The listing builds one solid part. Answer for the finished solid, in the listing's coordinates (mm). A direction names the side the tool comes from. Give positions to 0.01 mm unless a question says otherwise; leave off trailing zeros. Loops run counter-clockwise (first coordinate to the right, second up) from the corner with the lowest first, then second, coordinate; pieces in that order, holes last. Notation, with made-up numbers: M -9,73 L 1,73 A34 cw 1,107 Z; hole C 42,88 d9. An arc over 180 degrees is marked long. Use one line per item in the form item = value. Start each with the question number.
1. The part is cut by section A-A (x = 402.5). Write down the section's boundary in (y, z), and give its area (3 significant figures).
2. Straight lines are drawn through the part: line 1 (X direction, y = 24.15, z = 0); line 2 (Z direction, x = 27, y = 1); line 3 (Z direction, x = -320, y = -2.5). For each, find the intervals that lie inside material, in ascending order. Write a range as from..to.
3. Each of these flat-tipped pins is pushed along its axis until it touches: pin 1 Ø3 at (x, z) = (-263.5, -5) entering from +Y; pin 2 Ø10.5 at (x, y) = (167, -2) entering from +Z; pin 3 Ø4 at (x, z) = (342.5, 10.5) entering from +Y. Where does it stop, or does it pass through?
4. The mould has two halves that part along Y. Classify faces 1 (the face through (-515, -13, -20)), 2 (the face through (7.2, -22.2, -11.5)), 3 (the face through (165.63, 6.31, -20.03)): released by +Y, released by -Y, zero draft, split by the parting line, or undercut.
5. For faces 4 (the face through (515, -13, -20)), 5 (the face through (120, -19, -10)), 6 (the face through (210, -19, -10)), determine the directions among +Z, -Z, +X, -X, +Y, -Y from which every point of the face is accessible in a straight line to the end or side of a thin tool.
from build123d import *

# Parameters (mm, degrees)
SKETCH1_R                     = 25
SKETCH1_R_2                   = 23
EXTRUDE_THIN1_DEPTH           = 515
EXTRUDE_THIN2_START           = 210
SKETCH1_3_R                   = 25
SKETCH1_3_R_2                 = 21
EXTRUDE_THIN2_DEPTH           = 90
CUT_EXTRUDE1_START            = 24.54
CUT_EXTRUDE1_DEPTH            = 492.672165684
CUT_EXTRUDE2_START            = -24.54
CUT_EXTRUDE2_DEPTH            = 492.672165793
CUT_EXTRUDE3_START            = -24.54
CUT_EXTRUDE3_DEPTH            = 492.672165793
CUT_EXTRUDE4_START            = 24.54
CUT_EXTRUDE4_DEPTH            = 492.672165793
M_0_295_DIAMETER_HOLE3_REACH  = 519.981
M_0_295_DIAMETER_HOLE3_BORE_R = 3.7465
M_0_295_DIAMETER_HOLE4_REACH  = 519.981
M_0_295_DIAMETER_HOLE4_BORE_R = 3.7465
M_0_295_DIAMETER_HOLE5_REACH  = 519.981
M_0_295_DIAMETER_HOLE5_BORE_R = 3.7465
M_0_295_DIAMETER_HOLE6_REACH  = 519.981
M_0_295_DIAMETER_HOLE6_BORE_R = 3.7465
CHAMFER1_SIZE                 = 0.5


with BuildPart() as part:
    # Sketch1 → Extrude-Thin1 (new, symmetric)
    with BuildSketch(Plane(origin=(0, 0, 0), x_dir=(0, 0, -1), z_dir=(1, 0, 0))):
        Circle(SKETCH1_R)
        Circle(SKETCH1_R_2, mode=Mode.SUBTRACT)
    extrude(amount=EXTRUDE_THIN1_DEPTH, both=True)

    # Sketch1<3> → Extrude-Thin2 (add)
    with BuildSketch(Plane(origin=(0, 0, 0), x_dir=(0, 0, -1), z_dir=(1, 0, 0)).offset(EXTRUDE_THIN2_START)):
        Circle(SKETCH1_3_R)
        Circle(SKETCH1_3_R_2, mode=Mode.SUBTRACT)
    extrude(amount=-EXTRUDE_THIN2_DEPTH)

    # Sketch3 → Cut-Extrude1 (cut, through all)
    with BuildSketch(Plane(origin=(0, 0, 0), x_dir=(1, 0, 0), z_dir=(0, 1, 0)).offset(CUT_EXTRUDE1_START)):
        with BuildLine():
            Line((-491.7775, -17.4725), (-458.1225, -17.4725))
            ThreePointArc((-458.1225, -17.4725), (-440.65, 0), (-458.1225, 17.4725))
            Line((-458.1225, 17.4725), (-491.7775, 17.4725))
            ThreePointArc((-491.7775, 17.4725), (-509.25, 0), (-491.7775, -17.4725))
        make_face()
    extrude(amount=CUT_EXTRUDE1_DEPTH, mode=Mode.SUBTRACT)

    # Sketch8 → Cut-Extrude2 (cut, through all)
    with BuildSketch(Plane.XY.offset(CUT_EXTRUDE2_START)):
        with BuildLine():
            Line((-272.5275, -17.4725), (-238.8725, -17.4725))
            ThreePointArc((-238.8725, -17.4725), (-221.4, 0), (-238.8725, 17.4725))
            Line((-238.8725, 17.4725), (-272.5275, 17.4725))
            ThreePointArc((-272.5275, 17.4725), (-290, 0), (-272.5275, -17.4725))
        make_face()
    extrude(amount=-CUT_EXTRUDE2_DEPTH, mode=Mode.SUBTRACT)

    # Sketch3<3> → Cut-Extrude3 (cut, through all)
    with BuildSketch(Plane(origin=(0, 0, 0), x_dir=(1, 0, 0), z_dir=(0, 1, 0)).offset(CUT_EXTRUDE3_START)):
        with BuildLine():
            ThreePointArc((458.1225, -17.4725), (440.65, 0), (458.1225, 17.4725))
            Line((458.1225, 17.4725), (491.7775, 17.4725))
            ThreePointArc((491.7775, 17.4725), (509.25, 0), (491.7775, -17.4725))
            Line((491.7775, -17.4725), (458.1225, -17.4725))
        make_face()
    extrude(amount=-CUT_EXTRUDE3_DEPTH, mode=Mode.SUBTRACT)

    # Sketch8<4> → Cut-Extrude4 (cut, through all)
    with BuildSketch(Plane.XY.offset(CUT_EXTRUDE4_START)):
        with BuildLine():
            Line((143.8725, -17.4725), (177.5275, -17.4725))
            ThreePointArc((177.5275, -17.4725), (195, 0), (177.5275, 17.4725))
            Line((177.5275, 17.4725), (143.8725, 17.4725))
            ThreePointArc((143.8725, 17.4725), (126.4, 0), (143.8725, -17.4725))
        make_face()
    extrude(amount=CUT_EXTRUDE4_DEPTH, mode=Mode.SUBTRACT)

    # M (0.295) Diameter Hole3 bore → M (0.295) Diameter Hole3 (cut, up to next)
    with BuildSketch(Plane(origin=(0, 24.54, 0), x_dir=(1, 0, 0), z_dir=(0, 1, 0)), mode=Mode.PRIVATE) as m_0_295_diameter_hole3_sk1:
        with Locations((-491.7775, 0)):
            Circle(M_0_295_DIAMETER_HOLE3_BORE_R)
    m_0_295_diameter_hole3_tool1 = extrude(m_0_295_diameter_hole3_sk1.sketch, amount=-M_0_295_DIAMETER_HOLE3_REACH, mode=Mode.PRIVATE) & part.part
    # M (0.295) Diameter Hole3 bore → M (0.295) Diameter Hole3 (cut, up to next)
    with BuildSketch(Plane(origin=(0, 24.54, 0), x_dir=(1, 0, 0), z_dir=(0, 1, 0)), mode=Mode.PRIVATE) as m_0_295_diameter_hole3_sk2:
        with Locations((-458.1225, 0)):
            Circle(M_0_295_DIAMETER_HOLE3_BORE_R)
    m_0_295_diameter_hole3_tool2 = extrude(m_0_295_diameter_hole3_sk2.sketch, amount=-M_0_295_DIAMETER_HOLE3_REACH, mode=Mode.PRIVATE) & part.part
    add(m_0_295_diameter_hole3_tool1.solids().sort_by_distance((-491.7775, 24.54, 0))[0], mode=Mode.SUBTRACT)
    add(m_0_295_diameter_hole3_tool2.solids().sort_by_distance((-458.1225, 24.54, 0))[0], mode=Mode.SUBTRACT)

    # M (0.295) Diameter Hole4 bore → M (0.295) Diameter Hole4 (cut, up to next)
    with BuildSketch(Plane(origin=(0, 0, -24.54), x_dir=(-1, 0, 0), z_dir=(0, 0, -1)), mode=Mode.PRIVATE) as m_0_295_diameter_hole4_sk1:
        with Locations((238.8725, 0)):
            Circle(M_0_295_DIAMETER_HOLE4_BORE_R)
    m_0_295_diameter_hole4_tool1 = extrude(m_0_295_diameter_hole4_sk1.sketch, amount=-M_0_295_DIAMETER_HOLE4_REACH, mode=Mode.PRIVATE) & part.part
    # M (0.295) Diameter Hole4 bore → M (0.295) Diameter Hole4 (cut, up to next)
    with BuildSketch(Plane(origin=(0, 0, -24.54), x_dir=(-1, 0, 0), z_dir=(0, 0, -1)), mode=Mode.PRIVATE) as m_0_295_diameter_hole4_sk2:
        with Locations((272.5275, 0)):
            Circle(M_0_295_DIAMETER_HOLE4_BORE_R)
    m_0_295_diameter_hole4_tool2 = extrude(m_0_295_diameter_hole4_sk2.sketch, amount=-M_0_295_DIAMETER_HOLE4_REACH, mode=Mode.PRIVATE) & part.part
    add(m_0_295_diameter_hole4_tool1.solids().sort_by_distance((-238.8725, 0, -24.54))[0], mode=Mode.SUBTRACT)
    add(m_0_295_diameter_hole4_tool2.solids().sort_by_distance((-272.5275, 0, -24.54))[0], mode=Mode.SUBTRACT)

    # M (0.295) Diameter Hole5 bore → M (0.295) Diameter Hole5 (cut, up to next)
    with BuildSketch(Plane.XY.offset(24.54), mode=Mode.PRIVATE) as m_0_295_diameter_hole5_sk1:
        with Locations((143.8725, 0)):
            Circle(M_0_295_DIAMETER_HOLE5_BORE_R)
    m_0_295_diameter_hole5_tool1 = extrude(m_0_295_diameter_hole5_sk1.sketch, amount=-M_0_295_DIAMETER_HOLE5_REACH, mode=Mode.PRIVATE) & part.part
    # M (0.295) Diameter Hole5 bore → M (0.295) Diameter Hole5 (cut, up to next)
    with BuildSketch(Plane.XY.offset(24.54), mode=Mode.PRIVATE) as m_0_295_diameter_hole5_sk2:
        with Locations((160.7, 0)):
            Circle(M_0_295_DIAMETER_HOLE5_BORE_R)
    m_0_295_diameter_hole5_tool2 = extrude(m_0_295_diameter_hole5_sk2.sketch, amount=-M_0_295_DIAMETER_HOLE5_REACH, mode=Mode.PRIVATE) & part.part
    # M (0.295) Diameter Hole5 bore → M (0.295) Diameter Hole5 (cut, up to next)
    with BuildSketch(Plane.XY.offset(24.54), mode=Mode.PRIVATE) as m_0_295_diameter_hole5_sk3:
        with Locations((177.5275, 0)):
            Circle(M_0_295_DIAMETER_HOLE5_BORE_R)
    m_0_295_diameter_hole5_tool3 = extrude(m_0_295_diameter_hole5_sk3.sketch, amount=-M_0_295_DIAMETER_HOLE5_REACH, mode=Mode.PRIVATE) & part.part
    add(m_0_295_diameter_hole5_tool1.solids().sort_by_distance((143.8725, 0, 24.54))[0], mode=Mode.SUBTRACT)
    add(m_0_295_diameter_hole5_tool2.solids().sort_by_distance((160.7, 0, 24.54))[0], mode=Mode.SUBTRACT)
    add(m_0_295_diameter_hole5_tool3.solids().sort_by_distance((177.5275, 0, 24.54))[0], mode=Mode.SUBTRACT)

    # M (0.295) Diameter Hole6 bore → M (0.295) Diameter Hole6 (cut, up to next)
    with BuildSketch(Plane(origin=(0, -24.54, 0), x_dir=(-1, 0, 0), z_dir=(0, -1, 0)), mode=Mode.PRIVATE) as m_0_295_diameter_hole6_sk1:
        with Locations((-491.7775, 0)):
            Circle(M_0_295_DIAMETER_HOLE6_BORE_R)
    m_0_295_diameter_hole6_tool1 = extrude(m_0_295_diameter_hole6_sk1.sketch, amount=-M_0_295_DIAMETER_HOLE6_REACH, mode=Mode.PRIVATE) & part.part
    # M (0.295) Diameter Hole6 bore → M (0.295) Diameter Hole6 (cut, up to next)
    with BuildSketch(Plane(origin=(0, -24.54, 0), x_dir=(-1, 0, 0), z_dir=(0, -1, 0)), mode=Mode.PRIVATE) as m_0_295_diameter_hole6_sk2:
        with Locations((-458.1225, 0)):
            Circle(M_0_295_DIAMETER_HOLE6_BORE_R)
    m_0_295_diameter_hole6_tool2 = extrude(m_0_295_diameter_hole6_sk2.sketch, amount=-M_0_295_DIAMETER_HOLE6_REACH, mode=Mode.PRIVATE) & part.part
    add(m_0_295_diameter_hole6_tool1.solids().sort_by_distance((491.7775, -24.54, 0))[0], mode=Mode.SUBTRACT)
    add(m_0_295_diameter_hole6_tool2.solids().sort_by_distance((458.1225, -24.54, 0))[0], mode=Mode.SUBTRACT)

    # Chamfer1
    chamfer1_edges = [part.edges().sort_by_distance(p)[0] for p in [
        (-515, 0, 25),
        (-515, 0, 23),
        (515, 0, 25),
        (515, 0, 23),
    ]]
    chamfer(chamfer1_edges, length=CHAMFER1_SIZE)


solid = part.part
Derived:
q1.outline = C 0,0 d50; hole C 0,0 d46
q1.area = 302 mm2
q2.line_1 = -515..-495.52, -488.03..-461.87, -454.38..515
q2.line_2 = -24.98..-22.98, 22.98..24.98
q2.line_3 = -24.87..-22.86, 22.86..24.87
q3.pin_1 = 24.75
q3.pin_2 = 24.54
q3.pin_3 = 23.51
q4.face_1 = zero draft
q4.face_2 = split by the parting line
q4.face_3 = undercut
q5.face_4 = +Z, -Z, +X, +Y, -Y
q5.face_5 = -X
q5.face_6 = +X
